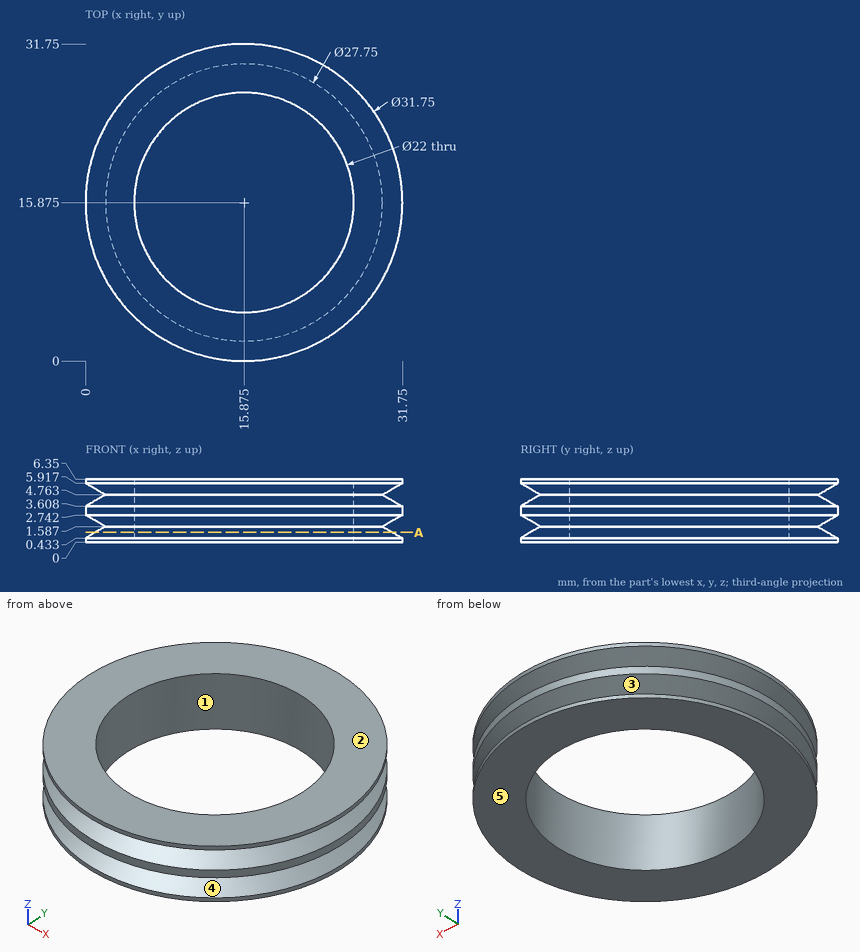
Job drawing, mm, ordinate dimensions from the low corner. One solid piece. A direction names the side the tool comes from. Round coordinates to 2 decimals unless told otherwise and drop trailing zeros. Loops run counter-clockwise (first coordinate to the right, second up) from the corner with the lowest first, then second, coordinate; pieces in that order, holes last. Notation, with made-up numbers: (87, 44) -> (142, 44) arc R12 ccw to (142, 67) -> close; hole circle Ø6 at (-21, -29). An arc over 180 degrees is marked (long way). Use a Markdown table: item, result.
1) Tool access for the marked faces 4 and 5: list every direction of +Z, -Z, +X, -X, +Y, -Y with a clear straight run to the whole face (end or side of a thin tool).
The answers:
| item | result |
|---|---|
| face 4 | none |
| face 5 | -Z, +X, -X, +Y, -Y |
2) Probe line 1 (X direction, y = 23, z = 0.75) (1 decimal); line 2 (Y direction, x = 12, z = 4.5) (1 decimal); line 3 (X direction, y = 24, z = 3) (1 decimal). List the from-to ranges inside material, lowest first. Write a range as [from, to].
The answers:
| item | result |
|---|---|
| line 1 | x = [2.3, 7.5], [24.3, 29.4] |
| line 2 | y = [2.1, 5.6], [26.2, 29.7] |
| line 3 | x = [2.2, 8.5], [23.3, 29.5] |
3) Pull direction Z, two halves, no side cores. Call the marked faces 1, 2 and 3: pulls with the +Z half, pulls with the -Z half, needs draft (parallel to the pull), parting line crosses it, or undercut.
The answers:
| item | result |
|---|---|
| face 1 | needs draft |
| face 2 | pulls with the +Z half |
| face 3 | undercut |
4) Drop flat-ended pins along their axis: pin 1 Ø3 at (x, z) = (27, 3.5) entering from -Y; pin 2 Ø5 at (x, y) = (10.5, 19) entering from +Z; pin 3 Ø3 at (y, z) = (9, 1) entering from -X. Give the stop position or say it passes through.
The answers:
| item | result |
|---|---|
| pin 1 | stops at y = 3.25 |
| pin 2 | passes through |
| pin 3 | stops at x = 0.98 |
5) Cut at A-A, the plane z = 1. List the corners of the cut face in (x, y) (1 decimal).
The answers:
| item | result |
|---|---|
| outline | circle Ø29.8 at (15.9, 15.9); hole circle Ø22 at (15.9, 15.9) |
